from build123d import *

# Parameters (mm, degrees)
BOSS_EXTRUDE1_DEPTH = 6


with BuildPart() as part:
    # Sketch1 → Boss-Extrude1 (new body)
    with BuildSketch(Plane.XZ):
        Polygon((48.466666667, 6), (48.466666667, 0), (69.2, 0), (69.2, 6), (90.933333333, 6), (90.933333333, 0), (111.666666667, 0), (111.666666667, 6), (133.4, 6), (133.4, 0), (154.133333333, 0), (154.133333333, 6), (175.866666667, 6), (175.866666667, 0), (196.6, 0), (196.6, 6), (218.333333333, 6), (218.333333333, 0), (239.066666667, 0), (239.066666667, 6), (260.8, 6), (260.8, 0), (281.533333333, 0), (281.533333333, 6), (303.266666667, 6), (303.266666667, 0), (324, 0), (324, 26.375), (330, 26.375), (330, 52.25), (324, 52.25), (324, 79.125), (330, 79.125), (330, 105), (0, 105), (0, 79.125), (6, 79.125), (6, 52.25), (0, 52.25), (0, 26.375), (6, 26.375), (6, 0), (26.733333333, 0), (26.733333333, 6), align=None)
    extrude(amount=-BOSS_EXTRUDE1_DEPTH)


solid = part.part
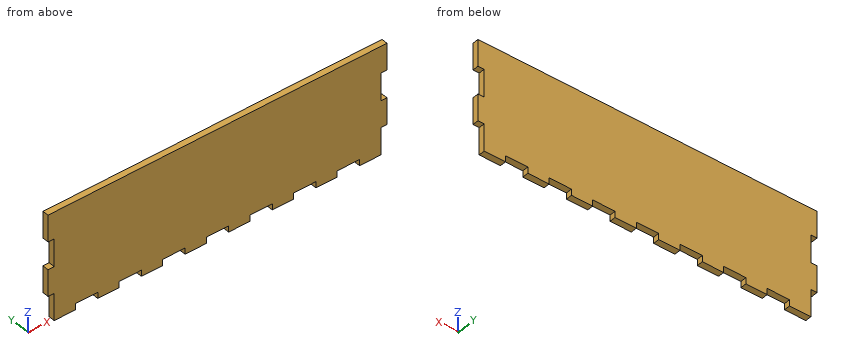
The model under review builds one solid part; all positions refer to its coordinate system, in mm. Round coordinates to 2 decimals unless told otherwise and drop trailing zeros. Write each loop counter-clockwise with the first axis right and the second up, starting at its lowest first coordinate (ties: lowest second). Pieces come first, ordered by that corner, then holes. Notation, with made-up numbers: (33.25, -18.5) -> (45.25, -18.5) arc R35 cw to (45.25, 18.5) -> close; hole circle Ø1 at (39.5, 69.5). An arc over 180 degrees is marked (long way). Answer as a JSON object with one key per item and string values.
1. We need section A-A on z = 68. State the section outline as (x, y) points, and give its area (3 significant figures).
Results found:
{"outline": "(6, 0) -> (324, 0) -> (324, 6) -> (6, 6) -> close", "area": "1,910 mm^2"}
2. To check wall thickness, follow line 1 along Z through (x, y) = (241.5, 1.95); line 2 along X through (y, z) = (4.75, 13.5). State the ranges of each line that lie inside material, in increasing order.
Results found:
{"line 1": "z = 6 to 105", "line 2": "x = 6 to 324"}
3. Clearance check with flat-ended pins moving along their axes: pin 1 (1.8 mm diameter, centred on y = 3.5, z = 4, fed in from -X); pin 2 (1.8 mm diameter, centred on y = 1.5, z = 3, fed in from +X); pin 3 (1.8 mm diameter, centred on x = 3, y = 4, fed in from -Z) (3 decimals). State where each tip first meets the part, or that it passes through.
Results found:
{"pin 1": "stops at x = 6", "pin 2": "stops at x = 324", "pin 3": "stops at z = 26.375"}
